Here's how the part is built. I have some questions about the finished solid (model axes, mm). A direction names the side the tool comes from. Round coordinates to 2 decimals unless told otherwise and drop trailing zeros. Order: outer loops, then holes, each group sorted by start corner. A loop starts at its lowest first (then second) coordinate and runs counter-clockwise, first axis right, second up. Notation, with made-up numbers: (35.25, -27) - (74.25, -27) arc R34 cw to (74.25, 11) - close; hole circle Ø9 at (-7, 37). An arc over 180 degrees is marked (long way). Answer as a JSON object with one key per item and string values.
```python
from build123d import *

# Parameters (mm, degrees)
SKETCH1_R                = 30.48
SKETCH1_R_2              = 24.13
BOSS_EXTRUDE1_DEPTH      = 152.4
BOSS_EXTRUDE2_REACH      = 190.508
BOSS_EXTRUDE2_END_RADIUS = 30.48
SKETCH2_R                = 30.48
SKETCH2_R_2              = 24.13


with BuildPart() as part:
    # Sketch1 → Boss-Extrude1 (new body)
    with BuildSketch(Plane.XY):
        with Locations(Location((0, 0, 0), (0, 0, 180))):
            Circle(SKETCH1_R)
        with Locations(Location((0, 0, 0), (0, 0, 180))):
            Circle(SKETCH1_R_2, mode=Mode.SUBTRACT)
    extrude(amount=BOSS_EXTRUDE1_DEPTH)

    # Boss-Extrude2: up to this cylinder (the profile starts outside it)
    boss_extrude2_end = Plane(origin=(0, 0, 105.817895), z_dir=(0, 0, -1)) * Cylinder(BOSS_EXTRUDE2_END_RADIUS, 442.976, mode=Mode.PRIVATE)
    # Sketch2 → Boss-Extrude2 (add, up to the surface)
    with BuildSketch(Plane(origin=(76.2, 0, 0), x_dir=(0, 0, -1), z_dir=(1, 0, 0)), mode=Mode.PRIVATE) as boss_extrude2_sk1:
        with Locations((-76.2, 0)):
            Circle(SKETCH2_R)
        with Locations((-76.2, 0)):
            Circle(SKETCH2_R_2, mode=Mode.SUBTRACT)
    boss_extrude2_tool1 = extrude(boss_extrude2_sk1.sketch, amount=-BOSS_EXTRUDE2_REACH, mode=Mode.PRIVATE) - boss_extrude2_end
    add(boss_extrude2_tool1.solids().sort_by_distance((76.2, 0, 105.817895))[0])


solid = part.part
```
1. If I drill on L1, parallel to Y at x = 0, z = 74; L2, parallel to X at y = -22, z = 94; L3, parallel to X at y = 1, z = 100, over which ranges is the centre line in solid material (lowest first)? Write a range as [from, to].
Responses:
{"L1": "[-30.48, -24.13], [24.13, 30.48]", "L2": "[-21.1, -9.91], [9.91, 76.2]", "L3": "[-30.46, -24.11], [24.11, 30.46]"}
2. For faces 1 (the face through (-29.07, -9.16, 75.13)), 2 (the face through (23, 9, 152.4)), 3 (the face through (47.81, -14.68, 95.35)), which set-ups out of +Z, -Z, +X, -X, +Y, -Y let a thin tool reach every point of the face, with its end or its side?
Responses:
{"face 1": "none", "face 2": "+Z, +X, -X, +Y, -Y", "face 3": "+X"}
3. Thinking about a two-plate mould opening in Y: for faces 4 (the face through (47.1, 25.7, 59.81)), 5 (the face through (23, 9, 0)), 6 (the face through (-23.016, -7.248, 75.133)), which applies, pulls with the +Y half, pulls with the -Y half, needs draft (parallel to the pull), parting line crosses it, or undercut?
Responses:
{"face 4": "parting line crosses it", "face 5": "needs draft", "face 6": "undercut"}
4. For P1, Ø10, axis at y = 17, z = 119.5, coming from the -X side; P2, Ø1, axis at y = -12, z = 35, coming from the +X side; P3, Ø1.5, axis at y = 5, z = 16.5, coming from the +X side; P4, Ø5, axis at x = -5.5, y = -19, coming from the +Z side, each with a flat end and sliding along its axis, tell me the tip position at first contact or that it passes through.
Responses:
{"P1": "x = -28.02", "P2": "x = 28.23", "P3": "x = 30.18", "P4": "through"}
5. Imagine slicing it at A-A (y = 0). List the corners of the cut face in (x, z) for me.
Responses:
{"outline": "(-30.48, 0) - (-24.13, 0) - (-24.13, 152.4) - (-30.48, 152.4) - close; (24.13, 0) - (30.48, 0) - (30.48, 45.72) - (76.2, 45.72) - (76.2, 52.07) - (30.48, 52.07) - (30.48, 100.33) - (76.2, 100.33) - (76.2, 106.68) - (30.48, 106.68) - (30.48, 152.4) - (24.13, 152.4) - close"}
6. Imagine slicing it at B-B (z = 76.2). List the corners of the cut face in (x, y) for me.
Responses:
{"outline": "(0, -30.48) - (76.2, -30.48) - (76.2, -24.13) - (18.62, -24.13) arc R30.48 ccw to (18.62, 24.13) - (76.2, 24.13) - (76.2, 30.48) - (0, 30.48) arc R30.48 ccw to start; hole circle Ø48.26 at (0, 0)"}
7. Imagine slicing it at C-C (x = -6). List the corners of the cut face in (y, z) for me.
Responses:
{"outline": "(-29.88, 0) - (-23.37, 0) - (-23.37, 152.4) - (-29.88, 152.4) - close; (23.37, 0) - (29.88, 0) - (29.88, 152.4) - (23.37, 152.4) - close"}
8. Imagine slicing it at D-D (y = -17). List the corners of the cut face in (x, z) for me.
Responses:
{"outline": "(-25.3, 0) - (-17.12, 0) - (-17.12, 152.4) - (-25.3, 152.4) - close; (17.12, 0) - (25.3, 0) - (25.3, 50.9) - (76.2, 50.9) - (76.2, 59.08) - (25.3, 59.08) - (25.3, 93.32) - (76.2, 93.32) - (76.2, 101.5) - (25.3, 101.5) - (25.3, 152.4) - (17.12, 152.4) - close"}
